from build123d import *

# Parameters (mm, degrees)
F0_W      = 63
F0_H      = 63
F1_DEPTH  = 32
F2_SIZE   = 4
F3_SIZE   = 2
F4_T      = -2
F5_W      = 55
F5_H      = 26.2
F6_DEPTH  = 1.5
F7_SIZE   = 1.49999
F8_R      = 8.132
F9_DEPTH  = 3.5
F10_W     = 14
F10_H     = 8
F11_DEPTH = 2
F13_W     = 14
F13_H     = 8
F14_DEPTH = 2
F15_SIZE  = 2
F16_SIZE  = 1.5
F18_DEPTH = 9.9
F19_DEPTH = 11


# Not quite as in the source:
# - a fillet or chamfer is up to 0.001 mm smaller than in the source, because OpenCascade refuses the exact size
# - a pattern or mirror of a feature is missing from the dataset's text; its kind, count and spacing are read off the source's solid


with BuildPart() as f1:
    # F0 (on Top) → F1 (new body)
    with BuildSketch(Plane.XY):
        with Locations((31.5, 31.5)):
            Rectangle(F0_W, F0_H)
    extrude(amount=F1_DEPTH)

    # F2
    f2_edges = [f1.edges().sort_by_distance(p)[0] for p in [
        (63, 0, 16),
        (63, 63, 16),
        (0, 0, 16),
        (0, 63, 16),
    ]]
    chamfer(f2_edges, length=F2_SIZE)

    # F3
    f3_edges = [f1.edges().sort_by_distance(p)[0] for p in [
        (0, 31.5, 32),
        (2, 61, 32),
        (2, 2, 32),
        (31.5, 63, 32),
        (31.5, 0, 32),
        (61, 61, 32),
        (61, 2, 32),
        (63, 31.5, 32),
    ]]
    chamfer(f3_edges, length=F3_SIZE)

    # F4
    f4_openings = [f1.faces().sort_by_distance(p)[0] for p in [
        (31.5, 31.5, 0),
    ]]
    offset(amount=F4_T, openings=f4_openings)

    # F5 (on face) → F6 (join)
    with BuildSketch(Plane.XZ):
        with Locations((31.5, 16.9)):
            Rectangle(F5_W, F5_H)
    extrude(amount=F6_DEPTH)

    # F7 (size 1.5 in the source; OpenCascade refuses exactly that, so slightly less here)
    f7_edges = [f1.edges().sort_by_distance(p)[0] for p in [
        (31.5, -1.5, 30),
        (4, -1.5, 16.9),
        (59, -1.5, 16.9),
    ]]
    chamfer(f7_edges, length=F7_SIZE)

    # F8 (on face) → F9 (cut, through all)
    with BuildSketch(Plane.XZ.offset(1.5)):
        with Locations((18.269, 16.955)):
            Circle(F8_R)
        with Locations((44.731, 16.955)):
            Circle(F8_R)
    extrude(amount=-F9_DEPTH, mode=Mode.SUBTRACT)

    # F10 (on face) → F11 (join, through all)
    with BuildSketch(Plane.XZ):
        with Locations((11.5, -4)):
            Rectangle(F10_W, F10_H)
        with Locations((51.5, -4)):
            Rectangle(F10_W, F10_H)
    extrude(amount=-F11_DEPTH)

    # F13 (on face) → F14 (join)
    with BuildSketch(Plane(origin=(0, 63, 0), x_dir=(-1, 0, 0), z_dir=(0, 1, 0))):
        with Locations((-51.5, -4)):
            Rectangle(F13_W, F13_H)
        with Locations((-11.5, -4)):
            Rectangle(F13_W, F13_H)
    extrude(amount=-F14_DEPTH)

    # F15
    f15_edges = [f1.edges().sort_by_distance(p)[0] for p in [
        (4.5, 1, -8),
        (18.5, 1, -8),
        (44.5, 1, -8),
        (58.5, 1, -8),
        (18.5, 62, -8),
        (4.5, 62, -8),
        (58.5, 62, -8),
        (44.5, 62, -8),
    ]]
    chamfer(f15_edges, length=F15_SIZE)

    # F16
    f16_edges = [f1.edges().sort_by_distance(p)[0] for p in [
        (18.5, 62, 0),
        (18.5, 1, 0),
        (44.5, 1, 0),
        (44.5, 62, 0),
    ]]
    chamfer(f16_edges, length=F16_SIZE)

    # F17 (on mid) → F18 (join)
    with BuildSketch(Plane(origin=(0, 31.5, 0), x_dir=(-1, 0, 0), z_dir=(0, 1, 0))):
        Polygon((0, -2.6), (0, 0), (-2, 0), (-2, -8.4), (0, -8.4), (0, -7.9), align=None)
        Polygon((2.1, -4.2), (0, -2.6), (0, -7.9), (2.1, -6.3), align=None)
    f18 = extrude(amount=-F18_DEPTH)

    # F18_copies: F18 across plane
    add(f18.mirror(Plane(origin=(31.5, 0, 0), x_dir=(0, 0, 1), z_dir=(1, 0, 0))))

    # F19 (add): a face of the model
    f19_faces = [f1.faces().sort_by_distance(p)[0] for p in [
        (0.3995726496, 31.5, -4.5320512821),
    ]]
    f19 = extrude(f19_faces, amount=F19_DEPTH)

    # F19_copies: F19 across plane
    add(f19.mirror(Plane(origin=(31.5, 0, 0), x_dir=(0, 0, 1), z_dir=(1, 0, 0))))


solid = f1.part
Geometry check sheet. Reference: the model listing, model coordinates, mm. A direction names the side the tool comes from. Round coordinates to 2 decimals unless told otherwise and drop trailing zeros. Order: outer loops, then holes, each group sorted by start corner. A loop starts at its lowest first (then second) coordinate and runs counter-clockwise, first axis right, second up. Notation, with made-up numbers: (-12, 36) -> (29, 36) arc R8 ccw to (29, 50) -> close; hole circle Ø3 at (-22.5, 42). An arc over 180 degrees is marked (long way). Use one line per item in the form item = value.
1. Go/stop test with flat-tipped pins: pin 1 (5 mm diameter, centred on y = 50, z = 15, fed in from -X); pin 2 (1.6 mm diameter, centred on y = 62, z = -3, fed in from -X); pin 3 (1.2 mm diameter, centred on x = 63, z = -3, fed in from -Y). Record where each tip stops, or that it passes through.
Working result:
pin_1 = 0
pin_2 = 4.5
pin_3 = 21.6
2. Mould release check, pull along X, two halves, no side actions. Record for faces 1 (the face through (-1.04, 31.9, -7.11)), 2 (the face through (31, 32, 32)), 3 (the face through (32, 61, 11)), 4 (the face through (57.5, 62, -7)): pulls with the +X half, pulls with the -X half, needs draft (parallel to the pull), parting line crosses it, or undercut.
Working result:
face_1 = pulls with the -X half
face_2 = needs draft
face_3 = undercut
face_4 = pulls with the +X half
3. Set-up check for faces 5 (the face through (61, 31, 15)), 6 (the face through (0, 42.5, -4)), 7 (the face through (31, 1, 0)): record each of +Z, -Z, +X, -X, +Y, -Y from which the full face is reachable in a straight line by a thin tool's end or side.
Working result:
face_5 = -Z
face_6 = -Z, +X, -X, +Y
face_7 = -Z, +Y, -Y
4. Cross-section at C-C, the plane y = 26. Enter the section's corners in (x, z), plus the area to 3 significant figures.
Working result:
outline = (-2.1, -6.3) -> (0, -7.9) -> (0, -8.4) -> (2, -8.4) -> (2, 29.17) -> (2.83, 30) -> (60.17, 30) -> (61, 29.17) -> (61, -8.4) -> (63, -8.4) -> (63, -7.9) -> (65.1, -6.3) -> (65.1, -4.2) -> (63, -2.6) -> (63, 30) -> (61, 32) -> (2, 32) -> (0, 30) -> (0, -2.6) -> (-2.1, -4.2) -> close
area = 292 mm^2
5. Scan lines: line 1 along X through (y, z) = (51, 3); line 2 along Y through (x, z) = (43.5, 27). Record each from-to range of solid material in increasing order. Write a range as from..to.
Working result:
line_1 = 0..2, 61..63
line_2 = -1.5..2, 61..63
6. Cross-section at D-D, the plane y = 19. Enter the section's corners in (x, z).
Working result:
outline = (0, 0) -> (2, 0) -> (2, 29.17) -> (2.83, 30) -> (60.17, 30) -> (61, 29.17) -> (61, 0) -> (63, 0) -> (63, 30) -> (61, 32) -> (2, 32) -> (0, 30) -> close
